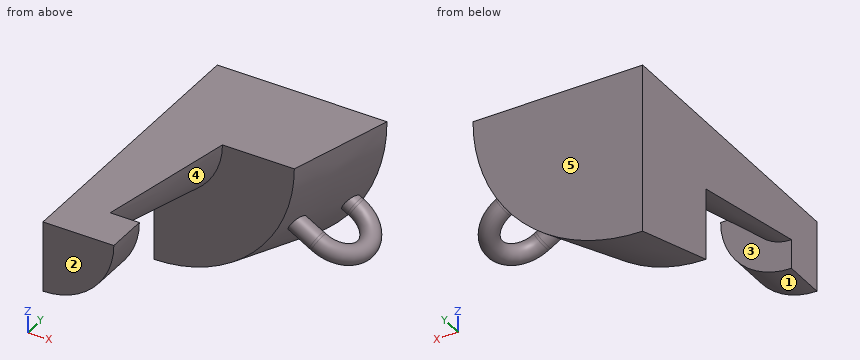
```python
from build123d import *
from build123d.topology import SkipClean

# Parameters (mm, degrees)
ROTATION1_ANGLE                 = 90
SKIZZE5_R                       = 3
SKIZZE7_R                       = 3
AUFSATZ_LINEAR_AUSTRAGEN1_DEPTH = 7.91623


with BuildPart() as part:
    # Skizze1 → Rotation1 (revolve)
    with BuildSketch(Plane.XY):
        Polygon((0, 0), (0, 91.42015625), (54.245597194, 91.42015625), (44.858528754, 58.217747507), (21.888186449, 58.217747507), (13.314555528, 13.381302083), (22.647732611, 13.381302083), (22.647732611, 0), align=None)
    revolve(axis=Axis((0, 0, 0), (0, 1, 0)), revolution_arc=ROTATION1_ANGLE)



with BuildPart() as body_2:
    # Austragung2: sweep along a path in Skizze6
    with BuildLine(Plane(origin=(0, 0, 0), x_dir=(0.866025404, 0, -0.5), z_dir=(0.5, 0, 0.866025404))) as austragung2_path:
        Line((54.245597194, 86.42015625), (55, 86.42015625))
        ThreePointArc((55, 86.42015625), (65, 76.42015625), (55, 66.42015625))
        Line((55, 66.42015625), (54.245597194, 66.42015625))
    # Skizze5 → Austragung2 (sweep)
    with BuildSketch(Plane(origin=(46.978065214, 0, -27.122798597), x_dir=(0.5, 0, 0.866025404), z_dir=(-0.866025404, 0, 0.5))):
        with Locations((0, 86.42015625)):
            Circle(SKIZZE5_R)
    sweep(path=austragung2_path.line)


with BuildPart() as part_1:
    with SkipClean():  # keep this step's faces unmerged: merging them makes the solid invalid here
        add(part.part)

        add(body_2.part)  # Aufsatz-Linear austragen1 merges body 2
        # Skizze7 → Aufsatz-Linear austragen1 (add)
        with BuildSketch(Plane(origin=(46.978065214, 0, -27.122798597), x_dir=(0.5, 0, 0.866025404), z_dir=(-0.866025404, 0, 0.5))):
            with Locations(Location((0, 66.42015625, 0), (0, 0, 190.622906641))):  # turned: the seam where the file's is
                Circle(SKIZZE7_R)
            with Locations(Location((0, 86.42015625, 0), (0, 0, 90))):  # turned: the seam where the file's is
                Circle(SKIZZE7_R)
        extrude(amount=AUFSATZ_LINEAR_AUSTRAGEN1_DEPTH)


solid = part_1.part
```
Work out the finished part from the listing and answer in its coordinate system (mm). Face numbers are marked on the shaded views. A direction names the side the tool comes from. Round coordinates to 2 decimals unless told otherwise and drop trailing zeros. Write each loop counter-clockwise with the first axis right and the second up, starting at its lowest first coordinate (ties: lowest second). Pieces come first, ordered by that corner, then holes. Notation, with made-up numbers: (-28.75, -4.5) - (28.25, -4.5) arc R10 cw to (28.25, 5.5) - close; hole circle Ø1 at (-22, 29). An arc over 180 degrees is marked (long way). Return JSON: item names as keys, results as strings. Group by question number.
Q1. This flat-tipped pin is pushed along its axis until it touches: pin 1 Ø1 at (y, z) = (79, -33) entering from +X. Where does it stop, or does it pass through?
Q2. Find the intervals of material crossed by L1, parallel to Y at x = 17.5, z = -18; L2, parallel to Z at x = 48, y = 85; L3, parallel to X at y = 76.5, z = -15.5, in increasing order.
Q3. For the marked faces 4 and 5, determine the directions among +Z, -Z, +X, -X, +Y, -Y from which every point of the face is accessible in a straight line to the end or side of a thin tool.
Q4. The mould has two halves that part along Y. Classify the marked faces 1, 2 and 3: released by +Y, released by -Y, zero draft, split by the parting line, or undercut.
Q5. The part is cut by section B-B on y = 34. Write down the section's boundary in (x, z), then the cut area to 3 significant figures.
Q6. The part is cut by section A-A on y = 9. Write down the section's boundary in (x, z), then the cut area to 3 significant figures.
Solved:
{
 "1": {"pin 1": "x = 59.11"},
 "2": {"L1": "58.22 to 91.42", "L2": "-30.89 to -24.66, -21.09 to 0", "L3": "0 to 47.57"},
 "3": {"face 4": "-Z, +X", "face 5": "+Z, -Z, +X, -X, +Y"},
 "4": {"face 1": "zero draft", "face 2": "released by -Y", "face 3": "undercut"},
 "5": {"outline": "(0, -17.26) arc R17.26 ccw to (17.26, 0) - (0, 0) - close", "area": "234 mm²"},
 "6": {"outline": "(0, -22.65) arc R22.65 ccw to (22.65, 0) - (0, 0) - close", "area": "403 mm²"}
}
